Verification items for the finished model (mm, model axes). Face numbers are marked on the shaded views. A direction names the side the tool comes from. Round coordinates to 2 decimals unless told otherwise and drop trailing zeros. Order: outer loops, then holes, each group sorted by start corner. A loop starts at its lowest first (then second) coordinate and runs counter-clockwise, first axis right, second up. Notation, with made-up numbers: M 69.25,86.5 L 97.25,86.5 A23 cw 97.25,106.5 Z; hole C 46.25,34.25 d10. An arc over 180 degrees is marked long. Return JSON: item names as keys, results as strings. Group by question number.
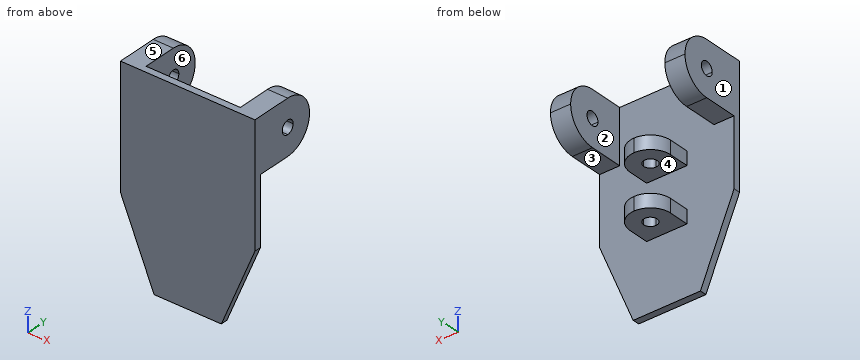
from build123d import *

# Parameters (mm, degrees)
EXTRUDE_1_DEPTH     = 10
EXTRUDE_2_DEPTH     = 200
SKETCH_3_W          = 140
SKETCH_3_H          = 100
CUT_EXTRUDE_1_DEPTH = 171
EXTRUDE_START       = -100
EXTRUDE_3_DEPTH     = 100
SKETCH_5_W          = 80
SKETCH_5_H          = 60
CUT_EXTRUDE_2_DEPTH = 110


with BuildPart() as part:
    # 草图1 → 凸台-拉伸1 (new body)
    with BuildSketch(Plane(origin=(0, 0, 0), x_dir=(1, 0, 0), z_dir=(0, 1, 0))):
        Polygon((-100, 0), (100, 0), (100, 180), (50, 300), (-50, 300), (-100, 180), align=None)
    extrude(amount=EXTRUDE_1_DEPTH)

    # 草图2 → 凸台-拉伸2 (add)
    with BuildSketch(Plane(origin=(100, 0, 0), x_dir=(0, 0, -1), z_dir=(1, 0, 0))):
        with BuildLine():
            ThreePointArc((80, 60), (68.284271247, 88.284271247), (40, 100))
            Line((40, 100), (40, 70))
            ThreePointArc((40, 70), (47.071067812, 67.071067812), (50, 60))
            ThreePointArc((50, 60), (47.071067812, 52.928932188), (40, 50))
            Line((40, 50), (40, 10))
            Line((40, 10), (80, 10))
            Line((80, 10), (80, 60))
        make_face()
        with BuildLine():
            Line((40, 70), (40, 100))
            ThreePointArc((40, 100), (11.715728753, 88.284271247), (0, 60))
            Line((0, 60), (0, 10))
            Line((0, 10), (40, 10))
            Line((40, 10), (40, 50))
            ThreePointArc((40, 50), (30, 60), (40, 70))
        make_face()
    extrude(amount=-EXTRUDE_2_DEPTH)

    # 草图3 → 切除-拉伸1 (cut)
    with BuildSketch(Plane(origin=(0, 10, 0), x_dir=(1, 0, 0), z_dir=(0, 1, 0))):
        with Locations((0, 50)):
            Rectangle(SKETCH_3_W, SKETCH_3_H)
    extrude(amount=CUT_EXTRUDE_1_DEPTH, mode=Mode.SUBTRACT)

    # 草图4 → 凸台-拉伸3 (add)
    with BuildSketch(Plane.XY.offset(EXTRUDE_START)):
        with BuildLine():
            Line((0, 30), (0, 10))
            Line((0, 10), (30, 10))
            Line((30, 10), (30, 40))
            ThreePointArc((30, 40), (21.213203436, 61.213203436), (0, 70))
            Line((0, 70), (0, 50))
            ThreePointArc((0, 50), (7.071067812, 47.071067812), (10, 40))
            ThreePointArc((10, 40), (7.071067812, 32.928932188), (0, 30))
        make_face()
        with BuildLine():
            Line((-30, 10), (0, 10))
            Line((0, 10), (0, 30))
            ThreePointArc((0, 30), (-10, 40), (0, 50))
            Line((0, 50), (0, 70))
            ThreePointArc((0, 70), (-21.213203436, 61.213203436), (-30, 40))
            Line((-30, 40), (-30, 10))
        make_face()
    extrude(amount=-EXTRUDE_3_DEPTH)

    # 草图5 → 切除-拉伸2 (cut)
    with BuildSketch(Plane(origin=(0, 10, 0), x_dir=(1, 0, 0), z_dir=(0, 1, 0))):
        with Locations((0, 150)):
            Rectangle(SKETCH_5_W, SKETCH_5_H)
    extrude(amount=CUT_EXTRUDE_2_DEPTH, mode=Mode.SUBTRACT)


solid = part.part
1. Cross-section at B-B (x = -6). Enter the section's corners in (y, z), plus the area to 3 significant figures.
2. Go/stop test with flat-tipped pins: pin 1 (15 mm diameter, centred on x = -87, y = 30, fed in from -Z); pin 2 (16 mm diameter, centred on y = 19, z = -186.5, fed in from +X); pin 3 (16 mm diameter, centred on y = 24, z = -189.5, fed in from -X); pin 4 (8 mm diameter, centred on x = -48, z = -167.5, fed in from -Y). Record where each tip stops, or that it passes through.
3. Cross-section at C-C (y = 36). Enter the section's corners in (x, z).
4. Draft check along Z on the marked faces 4, 5 and 6. Enter one of: +Z half, -Z half, draft (parallel to the pull), parting line (faces both ways), or undercut.
5. Cross-section at D-D (y = 81.5). Enter the section's corners in (x, z).
6. Access from +Z, -Z, +X, -X, +Y, -Y to the whole of each face (thin tool, end or side, straight path). Record for the marked faces 1, 2 and 3.
7. Cross-section at A-A (y = 22.5). Enter the section's corners in (x, z), plus the area to 3 significant figures.
8. Thickness scan on line 1 along X through (y, z) = (95.5, -34.5); line 2 along Z through (x, y) = (0, 52.5); line 3 along Z through (x, y) = (78.5, 60.5). Record the ranges inside material, lowest first. Write a range as from..to.
Computed:
{
 "1": {"outline": "M 0,-300 L 10,-300 L 10,-200 L 32,-200 L 32,-180 L 10,-180 L 10,-120 L 32,-120 L 32,-100 L 10,-100 L 10,0 L 0,0 Z; M 48,-200 L 69.39,-200 L 69.39,-180 L 48,-180 Z; M 48,-120 L 69.39,-120 L 69.39,-100 L 48,-100 Z", "area": "4,740 mm²"},
 "2": {"pin 1": "stops at z = -80", "pin 2": "stops at x = 30", "pin 3": "stops at x = -30", "pin 4": "stops at y = 0"},
 "3": {"outline": "M -100,-80 L -70,-80 L -70,0 L -100,0 Z; M -30,-200 L -9.17,-200 L -9.17,-180 L -30,-180 Z; M -30,-120 L -9.17,-120 L -9.17,-100 L -30,-100 Z; M 9.17,-200 L 30,-200 L 30,-180 L 9.17,-180 Z; M 9.17,-120 L 30,-120 L 30,-100 L 9.17,-100 Z; M 70,-80 L 100,-80 L 100,0 L 70,0 Z"},
 "4": {"face 4": "undercut", "face 5": "+Z half", "face 6": "draft"},
 "5": {"outline": "M -100,-73.73 L -70,-73.73 L -70,-6.27 L -100,-6.27 Z; M 70,-73.73 L 100,-73.73 L 100,-6.27 L 70,-6.27 Z"},
 "6": {"face 1": "+Z, -Z, -X, +Y, -Y", "face 2": "+Z, -Z, +Y", "face 3": "-Z, +X, -X, +Y"},
 "7": {"outline": "M -100,-80 L -70,-80 L -70,0 L -100,0 Z; M -30,-200 L 30,-200 L 30,-180 L -30,-180 Z; M -30,-120 L 30,-120 L 30,-100 L -30,-100 Z; M 70,-80 L 100,-80 L 100,0 L 70,0 Z", "area": "7,200 mm²"},
 "8": {"line 1": "x = -100..-70, 70..100", "line 2": "z = -200..-180, -120..-100", "line 3": "z = -80..-49.99, -30.01..0"}
}
